Design review of the part shown in the three views and the two pictorial views. Dimensions are in mm from the part's minimum x, y and z. Give positions to 0.01 mm unless a question says otherwise; leave off trailing zeros. Order: outer loops, then holes, each group sorted by start corner. A loop starts at its lowest first (then second) coordinate and runs counter-clockwise, first axis right, second up.
Item 1: Consider section D-D (z = 1.8). Give the boundary of the cut face in (x, y).
Item 2: For probe 1 along X at (y, z) = (4, 1.55); probe 2 along X at (y, z) = (21, 0.35); probe 3 along X at (y, z) = (9, 1.8), list the stretches that pass through material, from the lowest coordinate up.
Item 3: Consider section A-A (y = 12). Give the boundary of the cut face in (x, z), plus the area to 3 significant figures.
Item 4: Consider section B-B (x = 11). Give the boundary of the cut face in (y, z).
Item 5: Consider section C-C (y = 20.5). Give the boundary of the cut face in (x, z), plus the area to 3 significant figures.
Item 6: For P1, Ø1.5, axis at x = 34, z = 2.5, coming from the -Y side, flat-tipped, find the tip position at first contact; note if it passes through.
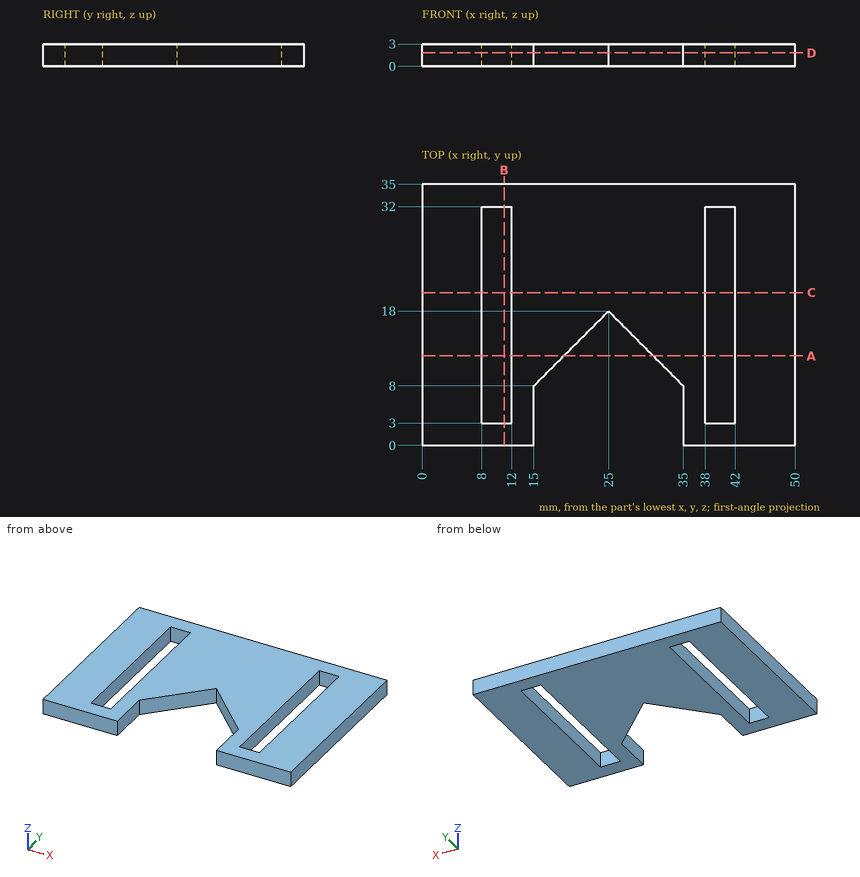
Resolved:
1. outline: (0, 0) - (15, 0) - (15, 8) - (25, 18) - (35, 8) - (35, 0) - (50, 0) - (50, 35) - (0, 35) - close; hole (8, 3) - (12, 3) - (12, 32) - (8, 32) - close; hole (38, 3) - (42, 3) - (42, 32) - (38, 32) - close
2. probe 1: x = 0 to 8, 12 to 15, 35 to 38, 42 to 50
2. probe 2: x = 0 to 8, 12 to 38, 42 to 50
2. probe 3: x = 0 to 8, 12 to 16, 34 to 38, 42 to 50
3. outline: (0, 0) - (8, 0) - (8, 3) - (0, 3) - close; (12, 0) - (19, 0) - (19, 3) - (12, 3) - close; (31, 0) - (38, 0) - (38, 3) - (31, 3) - close; (42, 0) - (50, 0) - (50, 3) - (42, 3) - close
3. area: 90.0 mm2
4. outline: (0, 0) - (3, 0) - (3, 3) - (0, 3) - close; (32, 0) - (35, 0) - (35, 3) - (32, 3) - close
5. outline: (0, 0) - (8, 0) - (8, 3) - (0, 3) - close; (12, 0) - (38, 0) - (38, 3) - (12, 3) - close; (42, 0) - (50, 0) - (50, 3) - (42, 3) - close
5. area: 126 mm2
6. P1: stops at y = 8.25
